For this review, use the dimensioned drawing (mm, ordinates from the lowest corner) and the shaded views. A direction names the side the tool comes from. Coordinates: 2 decimals unless noted, no trailing zeros. Write each loop counter-clockwise with the first axis right and the second up, starting at its lowest first coordinate (ties: lowest second). Pieces come first, ordered by that corner, then holes.
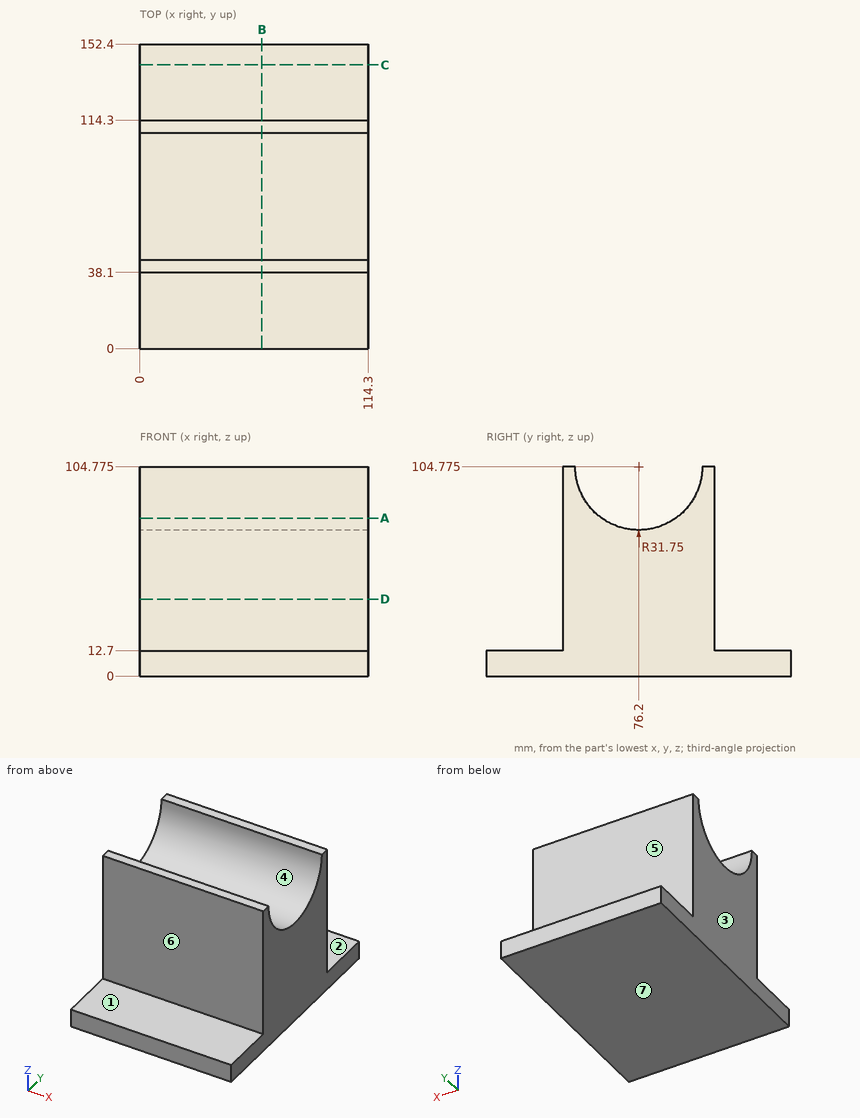
(1) Mouldability with a two-part tool opening along Y and no side actions: class the marked faces 4, 5, 6 and 7 as +Y half, -Y half, draft (parallel to the pull), parting line (faces both ways), or undercut.
(2) Wall thickness on line 1 (Z direction, x = 49.5, y = 19.5); line 2 (Y direction, x = 106.5, z = 69.5); line 3 (Y direction, x = 85, z = 84): over which ranges is each line inside the solid? List them lowest first.
(3) Insertion check: pin 1 Ø1.5 at (x, z) = (41.5, 61) entering from +Y; pin 2 Ø1.5 at (x, y) = (34, 16.5) entering from -Z; pin 3 Ø11.5 at (x, y) = (54, 137.5) entering from +Z; pin 4 Ø8 at (x, z) = (66.5, 65) entering from -Y. Each pin has a flat end and moves straight along its axis. Give the tip position at first contact, or say it passes through.
(4) Consider section D-D (z = 38.5). Give the boundary of the cut face in (x, y).
(5) For the marked faces 1, 2 and 3, list the 3-axis set-ups (+Z, -Z, +X, -X, +Y, -Y) from which the entire face can be reached by the end or side of a thin tool; tool diameter is ignored.
(6) Consider section B-B (x = 61). Give the boundary of the cut face in (y, z) (3 decimals).
(7) Consider section A-A (z = 79). Give the boundary of the cut face in (x, y).
(8) Consider section C-C (y = 142). Give the boundary of the cut face in (x, z), plus the area to 3 significant figures.
Results:
1. face 4: undercut
1. face 5: +Y half
1. face 6: -Y half
1. face 7: draft
2. line 1: z = 0 to 12.7
2. line 2: y = 38.1 to 114.3
2. line 3: y = 38.1 to 52.19, 100.21 to 114.3
3. pin 1: stops at y = 114.3
3. pin 2: stops at z = 0
3. pin 3: stops at z = 12.7
3. pin 4: stops at y = 38.1
4. outline: (0, 38.1) - (114.3, 38.1) - (114.3, 114.3) - (0, 114.3) - close
5. face 1: +Z, +X, -X, -Y
5. face 2: +Z, +X, -X, +Y
5. face 3: +Z, -Z, -X, +Y, -Y
6. outline: (0, 0) - (152.4, 0) - (152.4, 12.7) - (114.3, 12.7) - (114.3, 104.775) - (107.95, 104.775) arc R31.75 cw to (44.45, 104.775) - (38.1, 104.775) - (38.1, 12.7) - (0, 12.7) - close
7. outline: (0, 38.1) - (114.3, 38.1) - (114.3, 57.66) - (0, 57.66) - close; (0, 94.74) - (114.3, 94.74) - (114.3, 114.3) - (0, 114.3) - close
8. outline: (0, 0) - (114.3, 0) - (114.3, 12.7) - (0, 12.7) - close
8. area: 1,450 mm2
